```python
from build123d import *

# Parameters (mm, degrees)
BOSS_EXTRUDE1_DEPTH = 9.525
SKETCH2_R           = 4.23545
CUT_EXTRUDE1_DEPTH  = 4.7625


with BuildPart() as part:
    # Sketch1 → Boss-Extrude1 (new body)
    with BuildSketch(Plane(origin=(0, 0, 0), x_dir=(0, 0, -1), z_dir=(1, 0, 0))):
        Polygon((18.981321463, -8.05457391), (19.117264954, 7.726377291), (8.05457391, 18.981321463), (-7.726377291, 19.117264954), (-18.981321463, 8.05457391), (-19.117264954, -7.726377291), (-8.05457391, -18.981321463), (7.726377291, -19.117264954), align=None)
    extrude(amount=BOSS_EXTRUDE1_DEPTH)

    # Sketch2 → Cut-Extrude1 (cut)
    with BuildSketch(Plane.ZY):
        Circle(SKETCH2_R)
    extrude(amount=-CUT_EXTRUDE1_DEPTH, mode=Mode.SUBTRACT)


solid = part.part
```
Can you work these out from the model? Positions are in its coordinate system, mm. A direction names the side the tool comes from. Coordinates: 2 decimals unless noted, no trailing zeros. Loops run counter-clockwise (first coordinate to the right, second up) from the corner with the lowest first, then second, coordinate; pieces in that order, holes last. Notation, with made-up numbers: (79, 35) - (123, 35) arc R31 ccw to (123, 69) - close; hole circle Ø6 at (5.25, 71.5). An arc over 180 degrees is marked (long way). Use a Markdown table: item, result.
Item 1: If I drill on probe 1 along Y at (x, z) = (3.3, 0); probe 2 along Y at (x, z) = (1.25, 2); probe 3 along Z at (x, y) = (4.5, 3.5), over which ranges is the centre line in solid material (lowest first)? Write a range as from..to.
Numbers:
| item | result |
|---|---|
| probe 1 | y = -19.05..-4.24, 4.24..19.05 |
| probe 2 | y = -19.03..-3.73, 3.73..19.07 |
| probe 3 | z = -19.08..-2.39, 2.39..19.02 |
Item 2: For faces 1 (the face through (4.7, -13.28, 13.66)), 2 (the face through (2.35, -2.58, -3.36)), which set-ups out of +Z, -Z, +X, -X, +Y, -Y let a thin tool reach every point of the face, with its end or its side?
Numbers:
| item | result |
|---|---|
| face 1 | +Z, +X, -X, -Y |
| face 2 | -X |
Item 3: I want a section at D-D on z = -8.5. Please give me the cut outline in (x, y) (3 decimals), and give its area (3 significant figures).
Numbers:
| item | result |
|---|---|
| outline | (0, -18.357) - (9.525, -18.357) - (9.525, 18.528) - (0, 18.528) - close |
| area | 351 mm2 |
Item 4: I want a section at B-B on y = 0. Please give me the cut outline in (x, z) (1 decimal), and give its area (3 significant figures).
Numbers:
| item | result |
|---|---|
| outline | (0, -19.1) - (9.5, -19.1) - (9.5, 19.1) - (0, 19.1) - (0, 4.2) - (4.8, 4.2) - (4.8, -4.2) - (0, -4.2) - close |
| area | 323 mm2 |
Item 5: We'd pull the mould along Y, two halves only. Please class faces 3 (the face through (4.762, 0, 0)), 4 (the face through (4.7, 13.28, -13.66)), 5 (the face through (4.7, -13.66, -13.28)): released by +Y, released by -Y, zero draft, split by the parting line, or undercut.
Numbers:
| item | result |
|---|---|
| face 3 | undercut |
| face 4 | released by +Y |
| face 5 | released by -Y |
Item 6: Will these pins go through, and if not, where does the flat tip stop? pin 1 (2 mm diameter, centred on y = -14, z = 14, fed in from -X); pin 2 (1 mm diameter, centred on x = 5, z = -13.5, fed in from +Y); pin 3 (1 mm diameter, centred on x = 3, z = 0, fed in from -Y) (3 decimals); pin 4 (5 mm diameter, centred on x = 3.5, z = -11, fed in from +Y).
Numbers:
| item | result |
|---|---|
| pin 1 | stops at x = 0 |
| pin 2 | stops at y = 13.95 |
| pin 3 | stops at y = -19.055 |
| pin 4 | stops at y = 18.53 |
Item 7: I want a section at A-A on x = 2.5. Please give me the cut outline in (y, z).
Numbers:
| item | result |
|---|---|
| outline | (-19.12, -7.73) - (-8.05, -18.98) - (7.73, -19.12) - (18.98, -8.05) - (19.12, 7.73) - (8.05, 18.98) - (-7.73, 19.12) - (-18.98, 8.05) - close; hole circle Ø8.47 at (0, 0) |
Item 8: I want a section at C-C on x = 5.75. Please give me the cut outline in (y, z), and give its area (3 significant figures).
Numbers:
| item | result |
|---|---|
| outline | (-19.12, -7.73) - (-8.05, -18.98) - (7.73, -19.12) - (18.98, -8.05) - (19.12, 7.73) - (8.05, 18.98) - (-7.73, 19.12) - (-18.98, 8.05) - close |
| area | 1,200 mm2 |
